from build123d import *

# Parameters (mm, degrees)
SKETCH_1_W           = 200
SKETCH_1_H           = 100
EXTRUDE_2_DEPTH      = 60
SKETCH_4_W           = 96.5
SKETCH_4_H           = 42.3
CUT_EXTRUDE_7_DEPTH  = 180
SKETCH_10_R          = 2
CUT_EXTRUDE_12_DEPTH = 3
SKETCH_12_R          = 1
CUT_EXTRUDE_13_DEPTH = 3
SKETCH_16_R          = 29.5
CUT_EXTRUDE_14_DEPTH = 16
SKETCH_17_R          = 1.75
CUT_EXTRUDE_15_DEPTH = 10
SKETCH_22_R          = 4.000000002
CUT_EXTRUDE_16_DEPTH = 0.001
FILLET_1_R           = 10
FILLET_2_R           = 10
FILLET_3_R           = 10
FILLET_4_R           = 10


with BuildPart() as part:
    # 草图1 → 凸台-拉伸2 (new body)
    with BuildSketch(Plane(origin=(0, 0, 0), x_dir=(1, 0, 0), z_dir=(0, 1, 0))):
        Rectangle(SKETCH_1_W, SKETCH_1_H)
    extrude(amount=EXTRUDE_2_DEPTH)

    # 草图4 → 切除-拉伸7 (cut)
    with BuildSketch(Plane(origin=(0, 0, -50), x_dir=(-1, 0, 0), z_dir=(0, 0, -1))):
        with Locations((-50, 30)):
            Rectangle(SKETCH_4_W, SKETCH_4_H)
    extrude(amount=-CUT_EXTRUDE_7_DEPTH, mode=Mode.SUBTRACT)

    # 草图10 → 切除-拉伸12 (cut)
    with BuildSketch(Plane(origin=(0, 60, 0), x_dir=(1, 0, 0), z_dir=(0, 1, 0))):
        with Locations(Location((0, -41, 0), (0, 0, 270))):
            Circle(SKETCH_10_R)
    extrude(amount=-CUT_EXTRUDE_12_DEPTH, mode=Mode.SUBTRACT)

    # 草图12 → 切除-拉伸13 (cut)
    with BuildSketch(Plane(origin=(0, 0, -50), x_dir=(-1, 0, 0), z_dir=(0, 0, -1))):
        with Locations((0, 30)):
            Circle(SKETCH_12_R)
    extrude(amount=-CUT_EXTRUDE_13_DEPTH, mode=Mode.SUBTRACT)

    # 草图16 → 切除-拉伸14 (cut)
    with BuildSketch(Plane(origin=(0, 60, 0), x_dir=(1, 0, 0), z_dir=(0, 1, 0))):
        with Locations(Location((49.50076584, 0, 0), (0, 0, 270))):
            Circle(SKETCH_16_R)
    extrude(amount=-CUT_EXTRUDE_14_DEPTH, mode=Mode.SUBTRACT)

    # 草图17 → 切除-拉伸15 (cut)
    with BuildSketch(Plane(origin=(0, 8.85, 0), x_dir=(1, 0, 0), z_dir=(0, 1, 0))):
        with Locations(Location((50, -44.5, 0), (0, 0, 270))):
            Circle(SKETCH_17_R)
        with Locations(Location((18.533748237, -31.466251763, 0), (0, 0, 270))):
            Circle(SKETCH_17_R)
        with Locations(Location((5.5, 0, 0), (0, 0, 270))):
            Circle(SKETCH_17_R)
        with Locations(Location((18.533748237, 31.466251763, 0), (0, 0, 270))):
            Circle(SKETCH_17_R)
        with Locations(Location((50, 44.5, 0), (0, 0, 270))):
            Circle(SKETCH_17_R)
        with Locations(Location((81.466251763, 31.466251763, 0), (0, 0, 270))):
            Circle(SKETCH_17_R)
        with Locations(Location((94.5, 0, 0), (0, 0, 270))):
            Circle(SKETCH_17_R)
        with Locations(Location((81.466251763, -31.466251763, 0), (0, 0, 270))):
            Circle(SKETCH_17_R)
    extrude(amount=-CUT_EXTRUDE_15_DEPTH, mode=Mode.SUBTRACT)

    # 草图22 → 切除-拉伸16 (cut)
    with BuildSketch(Plane(origin=(0, 60, 0), x_dir=(1, 0, 0), z_dir=(0, 1, 0))):
        with Locations(Location((-39.943771533, -6.115069491, 0), (0, 0, 270))):
            Circle(SKETCH_22_R)
    extrude(amount=-CUT_EXTRUDE_16_DEPTH, mode=Mode.SUBTRACT)

    # 圆角1
    fillet_1_edges = [part.edges().sort_by_distance(p)[0] for p in [
        (-100, 30, -50),
    ]]
    fillet(fillet_1_edges, radius=FILLET_1_R)

    # 圆角2
    fillet_2_edges = [part.edges().sort_by_distance(p)[0] for p in [
        (-100, 30, 50),
    ]]
    fillet(fillet_2_edges, radius=FILLET_2_R)

    # 圆角3
    # the kernel refuses this fillet: 10 mm, written as the material it takes off along each edge
    with BuildSketch(Plane(origin=(100, -25, 50), x_dir=(-1, 0, 0), z_dir=(0, 1, 0))) as fillet_3_piece_1:
        with BuildLine():
            CenterArc((FILLET_3_R, -FILLET_3_R), FILLET_3_R, 90, 90)
            Line((0, -FILLET_3_R), (0, 0))
            Line((0, 0), (FILLET_3_R, 0))
        make_face()
    extrude(amount=110, mode=Mode.SUBTRACT)

    # 圆角4
    # the kernel refuses this fillet: 10 mm, written as the material it takes off along each edge
    with BuildSketch(Plane(origin=(100, -25, -50), x_dir=(0, 0, 1), z_dir=(0, 1, 0))) as fillet_4_piece_1:
        with BuildLine():
            CenterArc((FILLET_4_R, -FILLET_4_R), FILLET_4_R, 90, 90)
            Line((0, -FILLET_4_R), (0, 0))
            Line((0, 0), (FILLET_4_R, 0))
        make_face()
    extrude(amount=110, mode=Mode.SUBTRACT)


solid = part.part
Source: CAD feature listing. Evaluate the final solid. Frame: model axes, mm. A direction names the side the tool comes from. Round coordinates to 2 decimals unless told otherwise and drop trailing zeros. Loops run counter-clockwise (first coordinate to the right, second up) from the corner with the lowest first, then second, coordinate; pieces in that order, holes last.
Q1. Section A-A, the plane y = 15.5. Return loops of the section in (x, z), plus the area to 3 significant figures.
Q2. First-contact query: P1, Ø1.8, axis at x = 0, y = 30, coming from the -Z side; P2, Ø2, axis at x = 81.47, z = -31.47, coming from the -Y side. Flat tips, straight axial feed; report the tip coordinate or a pass-through.
Q3. Mould query, pull axis Z, two halves, no side actions, for faces 4 (the face through (51, 8.85, -1)), 5 (the face through (49.33, 4.487, -42.883)), 6 (the face through (-21, 30, 50)), 7 (the face through (18.611, 4.487, -33.215)). Classes: pulls with the +Z half, pulls with the -Z half, needs draft (parallel to the pull), parting line crosses it, or undercut.
Q4. Ray query, line 1 (X direction, y = 2, z = 0); line 2 (X direction, y = 43.5, z = -6); line 3 (Y direction, x = 87.5, z = 43.5). Return the intervals inside material, ascending.
Q5. Access query for faces 1 (the face through (1.75, 30, -1)), 2 (the face through (49.33, 4.487, 46.117)), 3 (the face through (0, 59, 39)). Directions: +Z, -Z, +X, -X, +Y, -Y. A direction counts if a zero-diameter tool reaches every point of the face in a straight line with its end or side. Return the directions, or none.
Q6. Section B-B, the plane z = -36. Return loops of the section in (x, y), plus the area to 3 significant figures.
Q7. Section D-D, the plane z = 17. Return loops of the section in (x, y).
Q8. Section C-C, the plane x = 43.5. Return loops of the section in (y, z).
Solutions:
1. outline: (-100, -40) arc R10 ccw to (-90, -50) - (1.75, -50) - (1.75, 50) - (-90, 50) arc R10 ccw to (-100, 40) - close; (98.25, -45.65) arc R10 ccw to (100, -40) - (100, 40) arc R10 ccw to (98.25, 45.65) - close
1. area: 10,300 mm2
2. P1: stops at z = -47
2. P2: stops at y = 51.15
3. face 4: needs draft
3. face 5: undercut
3. face 6: pulls with the +Z half
3. face 7: undercut
4. line 1: x = -100 to 3.75, 7.25 to 92.75, 96.25 to 100
4. line 2: x = -100 to 1.75, 98.25 to 100
4. line 3: y = 0 to 8.85, 51.15 to 60
5. face 1: +Z, -Z
5. face 2: -Y
5. face 3: +Y
6. outline: (-100, 0) - (100, 0) - (100, 60) - (-100, 60) - close; hole (1.75, 8.85) - (98.25, 8.85) - (98.25, 51.15) - (1.75, 51.15) - close
6. area: 7,920 mm2
7. outline: (-100, 0) - (100, 0) - (100, 60) - (73.61, 60) - (73.61, 51.15) - (98.25, 51.15) - (98.25, 8.85) - (1.75, 8.85) - (1.75, 51.15) - (25.39, 51.15) - (25.39, 60) - (-100, 60) - close
8. outline: (0, -50) - (8.85, -50) - (8.85, 50) - (0, 50) - close; (51.15, -50) - (60, -50) - (60, -28.88) - (51.15, -28.88) - close; (51.15, 28.88) - (60, 28.88) - (60, 50) - (51.15, 50) - close
